```python
from build123d import *

# Parameters (mm, degrees)
SKETCH_1_R          = 40
EXTRUDE_1_DEPTH     = 15
SKETCH_2_R          = 18
EXTRUDE_2_DEPTH     = 10
SKETCH_3_R          = 10
CUT_EXTRUDE_1_DEPTH = 81
SKETCH_4_W          = 6
SKETCH_4_H          = 13
CUT_EXTRUDE_2_DEPTH = 81
SKETCH_5_R          = 6
CUT_EXTRUDE_3_DEPTH = 62.846584384


with BuildPart() as part:
    # 草图1 → 凸台-拉伸1 (new body)
    with BuildSketch(Plane.XY):
        Circle(SKETCH_1_R)
    extrude(amount=EXTRUDE_1_DEPTH)

    # 草图2 → 凸台-拉伸2 (add)
    with BuildSketch(Plane.XY.offset(15)):
        with Locations((10, 0)):
            Circle(SKETCH_2_R)
    extrude(amount=EXTRUDE_2_DEPTH)

    # 草图3 → 切除-拉伸1 (cut, symmetric)
    with BuildSketch(Plane.XY.offset(25)):
        with Locations((10, 0)):
            Circle(SKETCH_3_R)
    extrude(amount=CUT_EXTRUDE_1_DEPTH, both=True, mode=Mode.SUBTRACT)

    # 草图4 → 切除-拉伸2 (cut, symmetric)
    with BuildSketch(Plane.XY.offset(25)):
        with Locations((10, 6.5)):
            Rectangle(SKETCH_4_W, SKETCH_4_H)
    extrude(amount=CUT_EXTRUDE_2_DEPTH, both=True, mode=Mode.SUBTRACT)

    # 草图5 → 切除-拉伸3 (cut, through all)
    with BuildSketch(Plane.XY):
        with Locations((-18, 14)):
            Circle(SKETCH_5_R)
        with Locations((-18, -14)):
            Circle(SKETCH_5_R)
    extrude(amount=CUT_EXTRUDE_3_DEPTH, mode=Mode.SUBTRACT)


solid = part.part
```
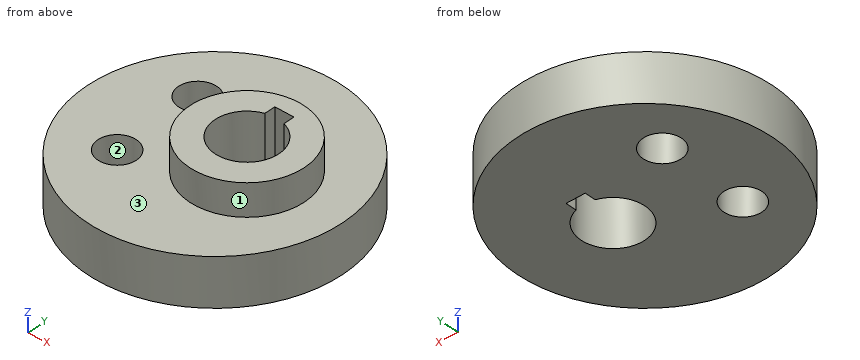
Could you check a few things on this model? Use its own coordinates, in mm. Face numbers are marked on the shaded views. Give positions to 0.01 mm unless a question says otherwise; leave off trailing zeros. Order: outer loops, then holes, each group sorted by start corner. A loop starts at its lowest first (then second) coordinate and runs counter-clockwise, first axis right, second up.
Q1. We'd pull the mould along X, two halves only. Please class the marked faces 1, 2 and 3: +X half, -X half, draft (parallel to the pull), parting line (faces both ways), or undercut.
Q2. Suppose I cut it at D-D, the plane z = 13.75. Write out the boundary of the cut face in (x, y).
Q3. I'm going to push flat-ended pins straight in: P1, Ø1.5, axis at x = 6, y = -26.5, coming from the -Z side; P2, Ø2, axis at x = 5.5, z = 17.5, coming from the -Y side; P3, Ø4, axis at x = 20, y = 20.5, coming from the +Z side; P4, Ø1.5, axis at x = 0, z = 16, coming from the -Y side. Where does each tip first touch, or does it pass through?
Q4. If I drill on line 1 along Y through (x, z) = (-20.5, 9); line 2 along Y through (x, z) = (-18, 4.5); line 3 along Z through (x, y) = (-21, 20), over which ranges is the centre line in solid material (lowest first)?
Q5. Suppose I cut it at C-C, the plane x = -16. Write out the boundary of the cut face in (y, z).
Q6. Suppose I cut it at A-A, the plane x = 10. Write out the boundary of the cut face in (y, z).
Q7. Suppose I cut it at B-B, the plane z = 19.5. Write out the boundary of the cut face in (x, y), and give its area (3 significant figures).
Solution:
1. face 1: parting line
1. face 2: undercut
1. face 3: draft
2. outline: circle Ø80 at (0, 0); hole circle Ø12 at (-18, -14); hole circle Ø12 at (-18, 14); hole (7, 9.54) arc R10 ccw (long way) to (13, 9.54) - (13, 13) - (7, 13) - close
3. P1: stops at z = 0
3. P2: stops at y = -17.66
3. P3: stops at z = 15
3. P4: stops at y = -15.44
4. line 1: y = -34.35 to -19.45, -8.55 to 8.55, 19.45 to 34.35
4. line 2: y = -35.72 to -20, -8 to 8, 20 to 35.72
4. line 3: z = 0 to 15
5. outline: (-36.66, 0) - (-19.66, 0) - (-19.66, 15) - (-36.66, 15) - close; (-8.34, 0) - (8.34, 0) - (8.34, 15) - (-8.34, 15) - close; (19.66, 0) - (36.66, 0) - (36.66, 15) - (19.66, 15) - close
6. outline: (-38.73, 0) - (-10, 0) - (-10, 25) - (-18, 25) - (-18, 15) - (-38.73, 15) - close; (13, 0) - (38.73, 0) - (38.73, 15) - (18, 15) - (18, 25) - (13, 25) - close
7. outline: circle Ø36 at (10, 0); hole (7, 9.54) arc R10 ccw (long way) to (13, 9.54) - (13, 13) - (7, 13) - close
7. area: 685 mm2
